Verification items for the finished model (mm, model axes). A direction names the side the tool comes from. Coordinates: 2 decimals unless noted, no trailing zeros. Write each loop counter-clockwise with the first axis right and the second up, starting at its lowest first coordinate (ties: lowest second). Pieces come first, ordered by that corner, then holes. Notation, with made-up numbers: (-1.5, 26) -> (14.5, 26) arc R24 ccw to (14.5, 60) -> close; hole circle Ø5 at (82.5, 41). An arc over 180 degrees is marked (long way). Use CSV: the item, a comma, the result in double quotes.
```python
from build123d import *

# Parameters (mm, degrees)
BOX004_W     = 10
BOX004_H     = 8
BOX004_DEPTH = 30
BOX003_W     = 10
BOX003_H     = 8
BOX003_DEPTH = 30
BOX001_W     = 75
BOX001_H     = 23
BOX001_DEPTH = 30
BOX002_W     = 81
BOX002_H     = 23
BOX002_DEPTH = 30
BOX_W        = 85
BOX_H        = 27
BOX_DEPTH    = 21
FILLET_R     = 0.4


with BuildPart() as cube004:
    # Box004 → Box004 (new body)
    with BuildSketch(Plane(origin=(80, 9.5, 2), x_dir=(1, 0, 0), z_dir=(0, 0, 1))):
        with Locations((5, 4)):
            Rectangle(BOX004_W, BOX004_H)
    extrude(amount=BOX004_DEPTH)


with BuildPart() as cube003:
    # Box003 → Box003 (new body)
    with BuildSketch(Plane(origin=(-2, 9.5, 5.5), x_dir=(1, 0, 0), z_dir=(0, 0, 1))):
        with Locations((5, 4)):
            Rectangle(BOX003_W, BOX003_H)
    extrude(amount=BOX003_DEPTH)


with BuildPart() as cube001:
    # Box001 → Box001 (new body)
    with BuildSketch(Plane(origin=(5, 2, 2), x_dir=(1, 0, 0), z_dir=(0, 0, 1))):
        with Locations((37.5, 11.5)):
            Rectangle(BOX001_W, BOX001_H)
    extrude(amount=BOX001_DEPTH)


with BuildPart() as cube002:
    # Box002 → Box002 (new body)
    with BuildSketch(Plane(origin=(2, 2, 5.5), x_dir=(1, 0, 0), z_dir=(0, 0, 1))):
        with Locations((40.5, 11.5)):
            Rectangle(BOX002_W, BOX002_H)
    extrude(amount=BOX002_DEPTH)


with BuildPart() as fillet_body:
    # Box → Box (new body)
    with BuildSketch(Plane.XY):
        with Locations((42.5, 13.5)):
            Rectangle(BOX_W, BOX_H)
    extrude(amount=BOX_DEPTH)

    # Cut: cut Cube002
    add(cube002.part, mode=Mode.SUBTRACT)

    # Cut001: cut Cube001
    add(cube001.part, mode=Mode.SUBTRACT)

    # Cut002: cut Cube003
    add(cube003.part, mode=Mode.SUBTRACT)

    # Cut003: cut Cube004
    add(cube004.part, mode=Mode.SUBTRACT)

    # Fillet
    fillet_edges = [fillet_body.edges().sort_by_distance(p)[0] for p in [
        (0, 4.75, 21),
        (0, 9.5, 13.25),
        (0, 13.5, 5.5),
        (0, 17.5, 13.25),
        (0, 22.25, 21),
        (0, 27, 10.5),
        (0, 13.5, 0),
        (0, 0, 10.5),
        (1, 9.5, 21),
        (2, 5.75, 21),
        (3.5, 2, 21),
        (42.5, 2, 21),
        (81.5, 2, 21),
        (83, 5.75, 21),
        (84, 9.5, 21),
        (85, 4.75, 21),
        (42.5, 0, 21),
        (2, 9.5, 13.25),
        (2, 17.5, 13.25),
        (1, 17.5, 21),
        (84, 17.5, 21),
        (83, 21.25, 21),
        (81.5, 25, 21),
        (42.5, 25, 21),
        (3.5, 25, 21),
        (2, 21.25, 21),
        (42.5, 27, 21),
        (85, 22.25, 21),
        (42.5, 27, 0),
        (85, 27, 10.5),
        (85, 13.5, 0),
        (42.5, 0, 0),
        (85, 0, 10.5),
        (83, 9.5, 13.25),
        (85, 9.5, 11.5),
        (81.5, 9.5, 5.5),
        (80, 9.5, 3.75),
        (85, 13.5, 2),
        (85, 17.5, 11.5),
        (5, 13.5, 5.5),
        (83, 17.5, 13.25),
        (81.5, 17.5, 5.5),
        (80, 17.5, 3.75),
        (5, 5.75, 5.5),
        (80, 5.75, 5.5),
        (5, 21.25, 5.5),
        (80, 21.25, 5.5),
    ]]
    fillet(fillet_edges, radius=FILLET_R)


solid = fillet_body.part
```
1) Scan lines: L1, parallel to Y at x = 43.5, z = 9; L2, parallel to Z at x = 19.5, y = 20.5; L3, parallel to X at y = 7.25, z = 6.25. Record each from-to range of solid material in increasing order.
Return value:
L1,"0 to 2, 25 to 27"
L2,"0 to 2"
L3,"0 to 2, 83 to 85"
2) Mould release check, pull along X, two halves, no side actions. Record for faces 1 (the flat face through (85, 19, 10)), 2 (the flat face through (42, 1, 21)), 3 (the flat face through (83, 21, 13)): released by +X, released by -X, zero draft, split by the parting line, or undercut.
Return value:
face 1,"released by +X"
face 2,"zero draft"
face 3,"undercut"
3) Cross-section at D-D (z = 3). Record the boundary of the cut face in (x, y), plus the area to 3 significant figures.
Return value:
outline,"(0, 0.4) arc R0.4 ccw to (0.4, 0) -> (84.6, 0) arc R0.4 ccw to (85, 0.4) -> (85, 9.1) arc R0.4 ccw to (84.6, 9.5) -> (80.4, 9.5) arc R0.4 ccw to (80, 9.1) -> (80, 2) -> (5, 2) -> (5, 25) -> (80, 25) -> (80, 17.9) arc R0.4 ccw to (80.4, 17.5) -> (84.6, 17.5) arc R0.4 ccw to (85, 17.9) -> (85, 26.6) arc R0.4 ccw to (84.6, 27) -> (0.4, 27) arc R0.4 ccw to (0, 26.6) -> close"
area,"530 mm2"
4) Cross-section at B-B (x = 68). Record the boundary of the cut face in (y, z).
Return value:
outline,"(0, 0.4) arc R0.4 ccw to (0.4, 0) -> (26.6, 0) arc R0.4 ccw to (27, 0.4) -> (27, 20.6) arc R0.4 ccw to (26.6, 21) -> (25.4, 21) arc R0.4 ccw to (25, 20.6) -> (25, 2) -> (2, 2) -> (2, 20.6) arc R0.4 ccw to (1.6, 21) -> (0.4, 21) arc R0.4 ccw to (0, 20.6) -> close"
5) Cross-section at A-A (z = 10.75). Record the boundary of the cut face in (x, y), plus the area to 3 significant figures.
Return value:
outline,"(0, 0.4) arc R0.4 ccw to (0.4, 0) -> (84.6, 0) arc R0.4 ccw to (85, 0.4) -> (85, 9.1) arc R0.4 ccw to (84.6, 9.5) -> (83.4, 9.5) arc R0.4 ccw to (83, 9.1) -> (83, 2) -> (2, 2) -> (2, 9.1) arc R0.4 ccw to (1.6, 9.5) -> (0.4, 9.5) arc R0.4 ccw to (0, 9.1) -> close; (0, 17.9) arc R0.4 ccw to (0.4, 17.5) -> (1.6, 17.5) arc R0.4 ccw to (2, 17.9) -> (2, 25) -> (83, 25) -> (83, 17.9) arc R0.4 ccw to (83.4, 17.5) -> (84.6, 17.5) arc R0.4 ccw to (85, 17.9) -> (85, 26.6) arc R0.4 ccw to (84.6, 27) -> (0.4, 27) arc R0.4 ccw to (0, 26.6) -> close"
area,"400 mm2"
6) Gauge pin test, flat ends, axial feed: pin 1 (4 mm diameter, centred on x = 55, y = 22, fed in from +Z); pin 2 (3.5 mm diameter, centred on x = 3.5, y = 15.5, fed in from +Z). Record the tip position at first contact, or that the pin passes through.
Return value:
pin 1,"z = 2"
pin 2,"z = 5.5"
7) Cross-section at C-C (y = 16.5). Record the boundary of the cut face in (x, z).
Return value:
outline,"(0, 0.4) arc R0.4 ccw to (0.4, 0) -> (84.6, 0) arc R0.4 ccw to (85, 0.4) -> (85, 1.6) arc R0.4 ccw to (84.6, 2) -> (5, 2) -> (5, 5.1) arc R0.4 ccw to (4.6, 5.5) -> (0.4, 5.5) arc R0.4 ccw to (0, 5.1) -> close"
8) Set-up check for faces 4 (the flat face through (84, 17.5, 9)), 5 (the flat face through (2, 21, 13)), 6 (the flat face through (42, 14, 0)): record each of +Z, -Z, +X, -X, +Y, -Y from which the full face is reachable in a straight line by a thin tool's end or side.
Return value:
face 4,"+Z, +X"
face 5,"+Z"
face 6,"-Z, +X, -X, +Y, -Y"
